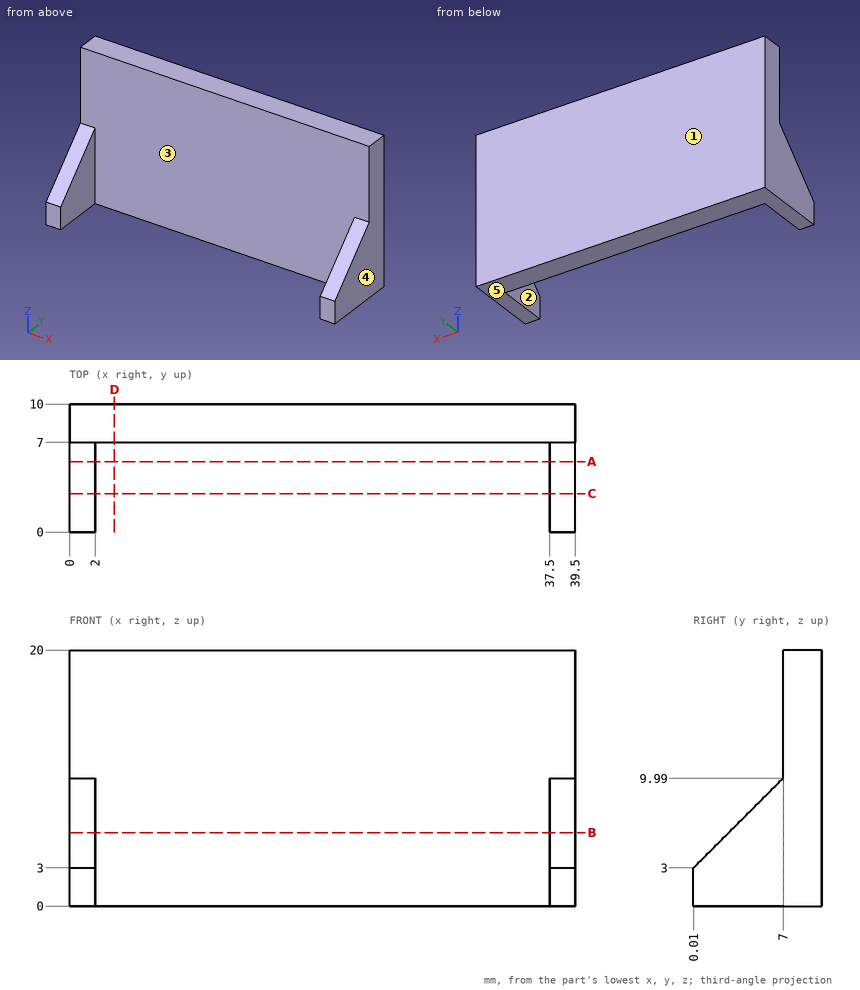
Job drawing, mm, ordinate dimensions from the low corner. One solid piece. A direction names the side the tool comes from. Give positions to 0.01 mm unless a question says otherwise; leave off trailing zeros. Loops run counter-clockwise (first coordinate to the right, second up) from the corner with the lowest first, then second, coordinate; pieces in that order, holes last. Notation, with made-up numbers: (72.5, 80) -> (94.5, 80) arc R20 ccw to (94.5, 84) -> close; hole circle Ø8 at (-9.5, 40.5). An arc over 180 degrees is marked (long way). Use a Markdown table: item, result. Add a question column.
(1) Slice it at A-A on y = 5.5. List the corners of the cut face in (x, z), and give its area (3 significant figures).
(2) Slice it at B-B on z = 5.75. List the corners of the cut face in (x, y).
(3) Drop a flat-ended pin along its axis: pin 1 Ø10 at (x, z) = (9.5, 8) entering from -Y. Give the stop position or say it passes through.
(4) Slice it at D-D on x = 3.5. List the corners of the cut face in (y, z), and give its area (3 significant figures).
(5) Wall check: line 1 along X through (y, z) = (5.5, 5); line 2 along Y through (x, z) = (2, 18.25). Give the ranges that are in metal, low to high.
(6) Tool access for the marked faces 1 and 2: list every direction of +Z, -Z, +X, -X, +Y, -Y with a clear straight run to the whole face (end or side of a thin tool).
(7) Mould opens along X. For the marked faces 3, 4 and 5 say: +X half, -X half, draft (parallel to the pull), parting line (faces both ways), or undercut.
(8) Slice it at C-C on y = 3. List the corners of the cut face in (x, z), and give its area (3 significant figures).
Filled sheet:
| question | item | result |
|---|---|---|
| 1 | outline | (0, 0) -> (2, 0) -> (2, 8.49) -> (0, 8.49) -> close; (37.5, 0) -> (39.5, 0) -> (39.5, 8.49) -> (37.5, 8.49) -> close |
| 1 | area | 34.0 mm2 |
| 2 | outline | (0, 2.76) -> (2, 2.76) -> (2, 7) -> (37.5, 7) -> (37.5, 2.76) -> (39.5, 2.76) -> (39.5, 10) -> (0, 10) -> close |
| 3 | pin 1 | y = 7 |
| 4 | outline | (7, 0) -> (10, 0) -> (10, 20) -> (7, 20) -> close |
| 4 | area | 60.0 mm2 |
| 5 | line 1 | 0 to 2, 37.5 to 39.5 |
| 5 | line 2 | 7 to 10 |
| 6 | face 1 | +Z, -Z, +X, -X, +Y |
| 6 | face 2 | +Z, -Z, -Y |
| 7 | face 3 | undercut |
| 7 | face 4 | +X half |
| 7 | face 5 | draft |
| 8 | outline | (0, 0) -> (2, 0) -> (2, 5.99) -> (0, 5.99) -> close; (37.5, 0) -> (39.5, 0) -> (39.5, 5.99) -> (37.5, 5.99) -> close |
| 8 | area | 24.0 mm2 |
